Read the model definition and answer for the solid it produces. Units are mm, in the model's axes. A direction names the side the tool comes from. Coordinates: 2 decimals unless noted, no trailing zeros. Loops run counter-clockwise (first coordinate to the right, second up) from the corner with the lowest first, then second, coordinate; pieces in that order, holes last. Notation, with made-up numbers: (65, -21) -> (91, -21) arc R17 ccw to (91, -2) -> close; hole circle Ø4 at (-24.75, 3). An arc over 180 degrees is marked (long way). Answer in a Markdown table with one row per item.
```python
from build123d import *

# Parameters (mm, degrees)
SKETCH1_W           = 50.8
SKETCH1_H           = 50.8
BOSS_EXTRUDE1_DEPTH = 406.4
SHELL1_T            = -1.5875
SKETCH2_R           = 12.7
CUT_EXTRUDE1_DEPTH  = 413.701150956


with BuildPart() as part:
    # Sketch1 → Boss-Extrude1 (new, symmetric)
    with BuildSketch(Plane(origin=(0, 0, 0), x_dir=(1, 0, 0), z_dir=(0, 1, 0))):
        with Locations((25.4, 25.4)):
            Rectangle(SKETCH1_W, SKETCH1_H)
    extrude(amount=BOSS_EXTRUDE1_DEPTH, both=True)

    # Shell1
    shell1_openings = [part.faces().sort_by_distance(p)[0] for p in [
        (25.4, 406.4, -25.4),
        (25.4, -406.4, -25.4),
    ]]
    offset(amount=SHELL1_T, openings=shell1_openings, kind=Kind.INTERSECTION)

    # Sketch2 → Cut-Extrude1 (cut, through all)
    with BuildSketch(Plane(origin=(50.8, 0, 0), x_dir=(0, 0, -1), z_dir=(1, 0, 0))):
        with Locations((25.4, 374.65)):
            Circle(SKETCH2_R)
    extrude(amount=-CUT_EXTRUDE1_DEPTH, mode=Mode.SUBTRACT)


solid = part.part
```
1. A cutting plane is placed at C-C on x = 38. Give the vertices of the cut face in (y, z).
A:
| item | result |
|---|---|
| outline | (-406.4, -50.8) -> (406.4, -50.8) -> (406.4, -49.21) -> (-406.4, -49.21) -> close; (-406.4, -1.59) -> (406.4, -1.59) -> (406.4, 0) -> (-406.4, 0) -> close |
2. A tool of negligible diameter and unlimited length cuts with its end or side. For faces 1 (the flat face through (0, 6, -25)), 2 (the flat face through (25, 6, -49.212)), from which of +Z, -Z, +X, -X, +Y, -Y can it reach the whole face along a straight path? Write none if from no direction.
A:
| item | result |
|---|---|
| face 1 | +Z, -Z, -X, +Y, -Y |
| face 2 | +Y, -Y |
3. A cutting plane is placed at D-D on y = 374.65. Give the vertices of the cut face in (x, z), and give its area (3 significant figures).
A:
| item | result |
|---|---|
| outline | (0, -50.8) -> (50.8, -50.8) -> (50.8, -38.1) -> (49.21, -38.1) -> (49.21, -49.21) -> (1.59, -49.21) -> (1.59, -38.1) -> (0, -38.1) -> close; (0, -12.7) -> (1.59, -12.7) -> (1.59, -1.59) -> (49.21, -1.59) -> (49.21, -12.7) -> (50.8, -12.7) -> (50.8, 0) -> (0, 0) -> close |
| area | 232 mm2 |
4. Find the intervals of material crossed by probe 1 along X at (y, z) = (-115, -25); probe 2 along Z at (x, y) = (17, -318); probe 3 along Y at (x, z) = (0.4, -25.4), in increasing order.
A:
| item | result |
|---|---|
| probe 1 | x = 0 to 1.59, 49.21 to 50.8 |
| probe 2 | z = -50.8 to -49.21, -1.59 to 0 |
| probe 3 | y = -406.4 to 361.95, 387.35 to 406.4 |
5. A cutting plane is placed at B-B on y = -281. Give the vertices of the cut face in (x, z).
A:
| item | result |
|---|---|
| outline | (0, -50.8) -> (50.8, -50.8) -> (50.8, 0) -> (0, 0) -> close; hole (1.59, -49.21) -> (49.21, -49.21) -> (49.21, -1.59) -> (1.59, -1.59) -> close |
6. The mould has two halves that part along Z. Classify faces 3 (the flat face through (25, 6, 0)), 4 (the flat face through (25, 6, -1.588)), 5 (the flat face through (23, 406.4, -1)): pulls with the +Z half, pulls with the -Z half, needs draft (parallel to the pull), parting line crosses it, or undercut.
A:
| item | result |
|---|---|
| face 3 | pulls with the +Z half |
| face 4 | undercut |
| face 5 | needs draft |
7. A cutting plane is placed at A-A on z = -25.4. Give the vertices of the cut face in (x, y).
A:
| item | result |
|---|---|
| outline | (0, -406.4) -> (1.59, -406.4) -> (1.59, 361.95) -> (0, 361.95) -> close; (0, 387.35) -> (1.59, 387.35) -> (1.59, 406.4) -> (0, 406.4) -> close; (49.21, -406.4) -> (50.8, -406.4) -> (50.8, 361.95) -> (49.21, 361.95) -> close; (49.21, 387.35) -> (50.8, 387.35) -> (50.8, 406.4) -> (49.21, 406.4) -> close |
